```python
from build123d import *

# Parameters (mm, degrees)
SKETCH1_W            = 150.1
SKETCH1_H            = 55.1
SKETCH1_R            = 1.5
BOSS_EXTRUDE1_DEPTH  = 1.7
SKETCH2_W            = 40.8
SKETCH2_H            = 2.5
BOSS_EXTRUDE2_DEPTH  = 2.4
SKETCH3_W            = 98
SKETCH3_H            = 60
SKETCH3_R            = 1.5
BOSS_EXTRUDE3_DEPTH  = 1.6
SKETCH4_W            = 98
SKETCH4_H            = 39.8
BOSS_EXTRUDE4_DEPTH  = 10
SKETCH5_W            = 75.5
SKETCH5_H            = 25.6
CUT_EXTRUDE1_DEPTH   = 0.8
SKETCH6_R            = 6
BOSS_EXTRUDE5_DEPTH  = 9.5
SKETCH7_W            = 6
SKETCH7_H            = 6
BOSS_EXTRUDE6_DEPTH  = 3
SKETCH8_R            = 1.75
BOSS_EXTRUDE7_DEPTH  = 1.7
SKETCH9_W            = 26.3
SKETCH9_H            = 26.5
BOSS_EXTRUDE8_DEPTH  = 2.8
SKETCH10_W           = 20.2
SKETCH10_H           = 8.6
BOSS_EXTRUDE9_DEPTH  = 9
SKETCH11_R           = 4.65
BOSS_EXTRUDE10_DEPTH = 9
SKETCH12_W           = 15
SKETCH12_H           = 12
BOSS_EXTRUDE11_DEPTH = 5.8
SKETCH13_R           = 3.4
BOSS_EXTRUDE12_DEPTH = 5.9
SKETCH14_R           = 7.5
BOSS_EXTRUDE13_DEPTH = 15


with BuildPart() as part:
    # Sketch1 → Boss-Extrude1 (new body)
    with BuildSketch(Plane(origin=(0, 0, 0), x_dir=(1, 0, 0), z_dir=(0, 1, 0))):
        Rectangle(SKETCH1_W, SKETCH1_H)
        with Locations(Location((-72.35, 24.85, 0), (0, 0, 270))):
            Circle(SKETCH1_R, mode=Mode.SUBTRACT)
        with Locations(Location((-72.35, -24.85, 0), (0, 0, 270))):
            Circle(SKETCH1_R, mode=Mode.SUBTRACT)
        with Locations(Location((72.35, 24.85, 0), (0, 0, 270))):
            Circle(SKETCH1_R, mode=Mode.SUBTRACT)
        with Locations(Location((72.35, -24.85, 0), (0, 0, 270))):
            Circle(SKETCH1_R, mode=Mode.SUBTRACT)
    extrude(amount=BOSS_EXTRUDE1_DEPTH)

    # Sketch2 → Boss-Extrude2 (add)
    with BuildSketch(Plane(origin=(0, 1.7, 0), x_dir=(1, 0, 0), z_dir=(0, 1, 0))):
        with Locations((-32.85, 21.9)):
            Rectangle(SKETCH2_W, SKETCH2_H)
    extrude(amount=BOSS_EXTRUDE2_DEPTH)

    # Sketch3 → Boss-Extrude3 (add)
    with BuildSketch(Plane(origin=(0, 4.1, 0), x_dir=(1, 0, 0), z_dir=(0, 1, 0))):
        with Locations((-12.55, -5.9)):
            Rectangle(SKETCH3_W, SKETCH3_H)
        with Locations(Location((-59.05, 21.6, 0), (0, 0, 270))):
            Circle(SKETCH3_R, mode=Mode.SUBTRACT)
        with Locations(Location((33.95, 21.6, 0), (0, 0, 270))):
            Circle(SKETCH3_R, mode=Mode.SUBTRACT)
        with Locations(Location((33.95, -33.4, 0), (0, 0, 270))):
            Circle(SKETCH3_R, mode=Mode.SUBTRACT)
        with Locations(Location((-59.05, -33.4, 0), (0, 0, 270))):
            Circle(SKETCH3_R, mode=Mode.SUBTRACT)
    extrude(amount=BOSS_EXTRUDE3_DEPTH)

    # Sketch4 → Boss-Extrude4 (add)
    with BuildSketch(Plane(origin=(0, 5.7, 0), x_dir=(1, 0, 0), z_dir=(0, 1, 0))):
        with Locations((-12.55, -5.9)):
            Rectangle(SKETCH4_W, SKETCH4_H)
    extrude(amount=BOSS_EXTRUDE4_DEPTH)

    # Sketch5 → Cut-Extrude1 (cut)
    with BuildSketch(Plane(origin=(0, 15.7, 0), x_dir=(1, 0, 0), z_dir=(0, 1, 0))):
        with Locations((-12.1, -6)):
            Rectangle(SKETCH5_W, SKETCH5_H)
    extrude(amount=-CUT_EXTRUDE1_DEPTH, mode=Mode.SUBTRACT)

    # Sketch6 → Boss-Extrude5 (add)
    with BuildSketch(Plane(origin=(0, 1.7, 0), x_dir=(1, 0, 0), z_dir=(0, 1, 0))):
        with Locations(Location((61.15, 16.95, 0), (0, 0, 90))):
            Circle(SKETCH6_R)
    extrude(amount=BOSS_EXTRUDE5_DEPTH)

    # Sketch7 → Boss-Extrude6 (add)
    with BuildSketch(Plane(origin=(0, 1.7, 0), x_dir=(1, 0, 0), z_dir=(0, 1, 0))):
        with Locations((61.85, -19.35)):
            Rectangle(SKETCH7_W, SKETCH7_H)
    extrude(amount=BOSS_EXTRUDE6_DEPTH)

    # Sketch8 → Boss-Extrude7 (add)
    with BuildSketch(Plane(origin=(0, 4.7, 0), x_dir=(1, 0, 0), z_dir=(0, 1, 0))):
        with Locations(Location((61.85, -19.35, 0), (0, 0, 270))):
            Circle(SKETCH8_R)
    extrude(amount=BOSS_EXTRUDE7_DEPTH)

    # Sketch9 → Boss-Extrude8 (add)
    with BuildSketch(Plane.XZ):
        with Locations((-61.9, 6)):
            Rectangle(SKETCH9_W, SKETCH9_H)
    extrude(amount=BOSS_EXTRUDE8_DEPTH)

    # Sketch10 → Boss-Extrude9 (add)
    with BuildSketch(Plane.XZ):
        with Locations((3.95, -1.35)):
            Rectangle(SKETCH10_W, SKETCH10_H)
        with Locations((-19.05, -1.35)):
            Rectangle(SKETCH10_W, SKETCH10_H)
    extrude(amount=BOSS_EXTRUDE9_DEPTH)

    # Sketch11 → Boss-Extrude10 (add)
    with BuildSketch(Plane.XZ):
        with Locations(Location((-62, -16.5, 0), (0, 0, 270))):
            Circle(SKETCH11_R)
    extrude(amount=BOSS_EXTRUDE10_DEPTH)

    # Sketch12 → Boss-Extrude11 (add)
    with BuildSketch(Plane(origin=(0, 1.7, 0), x_dir=(1, 0, 0), z_dir=(0, 1, 0))):
        with Locations((61.85, -2.05)):
            Rectangle(SKETCH12_W, SKETCH12_H)
    extrude(amount=BOSS_EXTRUDE11_DEPTH)

    # Sketch13 → Boss-Extrude12 (add)
    with BuildSketch(Plane(origin=(0, 7.5, 0), x_dir=(1, 0, 0), z_dir=(0, 1, 0))):
        with Locations(Location((62.05, -2.05, 0), (0, 0, 270))):
            Circle(SKETCH13_R)
    extrude(amount=BOSS_EXTRUDE12_DEPTH)

    # Sketch14 → Boss-Extrude13 (add)
    with BuildSketch(Plane(origin=(0, 13.4, 0), x_dir=(1, 0, 0), z_dir=(0, 1, 0))):
        with Locations(Location((62.05, -2.05, 0), (0, 0, 270))):
            Circle(SKETCH14_R)
    extrude(amount=BOSS_EXTRUDE13_DEPTH)


solid = part.part
```
Model file for the job. Use its own axes, mm. A direction names the side the tool comes from. Coordinates: 2 decimals unless noted, no trailing zeros. Write each loop counter-clockwise with the first axis right and the second up, starting at its lowest first coordinate (ties: lowest second). Pieces come first, ordered by that corner, then holes. Notation, with made-up numbers: (-24, 16.5) - (31, 16.5) arc R33 ccw to (31, 46.5) - close; hole circle Ø10 at (56.25, 5.5). An arc over 180 degrees is marked (long way). One line per item, written item: value. Start each with the question number.
1. Probe line 1 (Z direction, x = 72.35, y = 1.05); line 2 (X direction, y = 0.4, z = -24.85); line 3 (X direction, y = 4.4, z = 33.4). List the from-to ranges inside material, lowest first. Write a range as from..to.
2. Flat gauge pins, fed straight in: pin 1 (2 mm diameter, centred on x = -17, z = -19.5, fed in from +Y); pin 2 (8 mm diameter, centred on x = 7.5, y = 12.5, fed in from +Z); pin 3 (3 mm diameter, centred on x = 62, z = 20, fed in from +Y). Where does each tip first touch, or does it go through?
3. Slice it at D-D (z = 33.4). Write the cut outline in (x, y), plus the area to 3 significant figures.
4. Slice it at A-A (x = -3). Write the cut outline in (y, z).
5. Tool access for faces 4 (the flat face through (58.85, 3, 19)), 5 (the flat face through (-13, 15.7, -8)), 6 (the flat face through (62, 3, 22.35)), 7 (the flat face through (-62, -1, 19.25)), 8 (the flat face through (-13, 14.9, 6)): list every direction of +Z, -Z, +X, -X, +Y, -Y with a clear straight run to the whole face (end or side of a thin tool).
6. Slice it at C-C (x = -72.35). Write the cut outline in (y, z).
7. Slice it at B-B (z = 13.5). Write the cut outline in (x, y), plus the area to 3 significant figures.
8. Mould opens along Z. For faces 1 (the flat face through (-6.15, -4, -1)), 2 (the cylindrical face through (60.886, 6.384, -10.956)), 3 (the flat face through (-13, 11, 25.8)) say: released by +Z, released by -Z, zero draft, split by the parting line, or undercut.
Answers below:
1. line 1: z = -27.55..-26.35, -23.35..23.35, 26.35..27.55
1. line 2: x = -75.05..-73.85, -70.85..70.85, 73.85..75.05
1. line 3: x = -61.55..-60.55, -57.55..32.45, 35.45..36.45
2. pin 1: stops at y = 5.7
2. pin 2: stops at z = 25.8
2. pin 3: stops at y = 6.4
3. outline: (-61.55, 4.1) - (-60.55, 4.1) - (-60.55, 5.7) - (-61.55, 5.7) - close; (-57.55, 4.1) - (32.45, 4.1) - (32.45, 5.7) - (-57.55, 5.7) - close; (35.45, 4.1) - (36.45, 4.1) - (36.45, 5.7) - (35.45, 5.7) - close
3. area: 147 mm^2
4. outline: (-9, -5.65) - (0, -5.65) - (0, -27.55) - (1.7, -27.55) - (1.7, 27.55) - (0, 27.55) - (0, 2.95) - (-9, 2.95) - close; (4.1, -24.1) - (5.7, -24.1) - (5.7, -14) - (15.7, -14) - (15.7, -6.8) - (14.9, -6.8) - (14.9, 18.8) - (15.7, 18.8) - (15.7, 25.8) - (5.7, 25.8) - (5.7, 35.9) - (4.1, 35.9) - close
5. face 4: +Z, +Y
5. face 5: +Z, -Z, -X, +Y
5. face 6: +Z, +X, +Y
5. face 7: +Z, +X, -X, -Y
5. face 8: +Y
6. outline: (-2.8, -7.25) - (0, -7.25) - (0, -23.35) - (1.7, -23.35) - (1.7, 23.35) - (0, 23.35) - (0, 19.25) - (-2.8, 19.25) - close; (0, -27.55) - (1.7, -27.55) - (1.7, -26.35) - (0, -26.35) - close; (0, 26.35) - (1.7, 26.35) - (1.7, 27.55) - (0, 27.55) - close
7. outline: (-75.05, -2.8) - (-48.75, -2.8) - (-48.75, 0) - (75.05, 0) - (75.05, 1.7) - (-75.05, 1.7) - close; (-61.55, 4.1) - (36.45, 4.1) - (36.45, 15.7) - (25.65, 15.7) - (25.65, 14.9) - (-49.85, 14.9) - (-49.85, 15.7) - (-61.55, 15.7) - close
7. area: 1,410 mm^2
8. face 1: zero draft
8. face 2: undercut
8. face 3: released by +Z
